Autodesk Inventor part; units mm, degrees
ref_plane "YZ Plane" through (0, 0, 0) normal (1, 0, 0) x (0, 1, 0)
ref_plane "XZ Plane" through (0, 0, 0) normal (0, 1, 0) x (-1, 0, 0)
ref_plane "XY Plane" through (0, 0, 0) normal (0, 0, 1) x (1, 0, 0)
sketch "Sketch1" plane through (0, 0, 0) normal (0, 0, 1) x (1, 0, 0)
  line L0 (-22, 15) -> (-22, 8)
  line L1 (-21, 16) -> (-22, 15)
  line L2 (-12, 16) -> (-21, 16)
  line L3 (-11.8, 15.8) -> (-12, 16)
  arc A0 (-11.8, 15.8) -> (-11.0859, 15.5) centre (-11.0859, 16.5) ccw
  line L4 (-4.9141, 15.5) -> (-11.0859, 15.5)
  arc A1 (-4.9141, 15.5) -> (-4.2, 15.8) centre (-4.9141, 16.5) ccw
  line L5 (-4, 16) -> (-4.2, 15.8)
  line L6 (4, 16) -> (-4, 16)
  line L7 (4.2, 15.8) -> (4, 16)
  arc A2 (4.2, 15.8) -> (4.9141, 15.5) centre (4.9141, 16.5) ccw
  line L8 (11.0859, 15.5) -> (4.9141, 15.5)
  arc A3 (11.0859, 15.5) -> (11.8, 15.8) centre (11.0859, 16.5) ccw
  line L9 (12, 16) -> (11.8, 15.8)
  line L10 (21, 16) -> (12, 16)
  line L11 (22, 15) -> (21, 16)
  line L12 (22, 3) -> (22, 15)
  line L13 (21.5, 2.5) -> (22, 3)
  line L14 (21.5, -8) -> (21.5, 2.5)
  line L15 (20, -9.5) -> (21.5, -8)
  line L16 (9.45, -9.5) -> (20, -9.5)
  line L17 (6.6, -6.65) -> (9.45, -9.5)
  line L18 (6.6, -4.35) -> (6.6, -6.65)
  line L19 (7.7, -3.25) -> (6.6, -4.35)
  arc A4 (9.6, -1.075) -> (7.7, -3.25) centre (9.8292, -3.1926) ccw
  line L20 (10, -0.675) -> (9.6, -1.075)
  line L21 (10, 0.675) -> (10, -0.675)
  line L22 (9.6, 1.075) -> (10, 0.675)
  arc A5 (7.7, 3.1) -> (9.6, 1.075) centre (9.828, 3.1928) ccw
  line L23 (7.3, 3.5) -> (7.7, 3.1)
  line L24 (-7.3, 3.5) -> (7.3, 3.5)
  line L25 (-7.7, 3.1) -> (-7.3, 3.5)
  arc A6 (-9.6, 1.075) -> (-7.7, 3.1) centre (-9.828, 3.1928) ccw
  line L26 (-10, 0.675) -> (-9.6, 1.075)
  line L27 (-10, -0.675) -> (-10, 0.675)
  line L28 (-9.6, -1.075) -> (-10, -0.675)
  arc A7 (-7.7, -3.25) -> (-9.6, -1.075) centre (-9.8292, -3.1926) ccw
  line L29 (-6.6, -4.35) -> (-7.7, -3.25)
  line L30 (-6.6, -6.65) -> (-6.6, -4.35)
  line L31 (-9.45, -9.5) -> (-6.6, -6.65)
  line L32 (-20, -9.5) -> (-9.45, -9.5)
  line L33 (-21.5, -8) -> (-20, -9.5)
  line L34 (-21.5, 7.5) -> (-21.5, -8)
  line L35 (-22, 8) -> (-21.5, 7.5)
  point P0 (0, 0)
  point P1 (0, 0)
extrude "Extrusion1" add sketch "Sketch1" against normal blind 50.5
sketch "Sketch3" plane through (-21, 16, 0) normal (0, 1, 0) x (1, 0, 0)
  circle A0 centre (5.5, 41) radius 2.1
  circle A1 centre (36.5, 41) radius 2.1
  line L0 (9, 0) -> (0, 0)
  line L1 (9, 0) -> (9, 50.5)
  line L2 (0, 50.5) -> (9, 50.5)
  line L3 (0, 0) -> (0, 50.5)
  line L4 (42, 0) -> (33, 0)
  line L5 (42, 0) -> (42, 50.5)
  line L6 (33, 50.5) -> (42, 50.5)
  line L7 (33, 0) -> (33, 50.5)
  line L8 (42, 0) -> (33, 0)
  line L9 (4.5, 0) -> (4.5, 50.5) construction
  line L10 (0, 50.5) -> (9, 50.5)
  line L11 (0, 0) -> (0, 50.5)
  line L12 (0, 25.25) -> (42, 25.25) construction
  line L13 (42, 0) -> (42, 50.5)
  line L14 (21, 0) -> (21, 50.5) construction
  circle A2 centre (5.5, 9.5) radius 2.1
  circle A3 centre (36.5, 9.5) radius 2.1
  point P0 (19, 27.5)
  dimension "d5" = 31
  dimension "d6" = 4.2
  dimension "d7" = 15.75
extrude "Extrusion2" cut sketch "Sketch3" against normal blind 6 contours A0 | A1 | A2 | A3
properties part number "HGR20A"
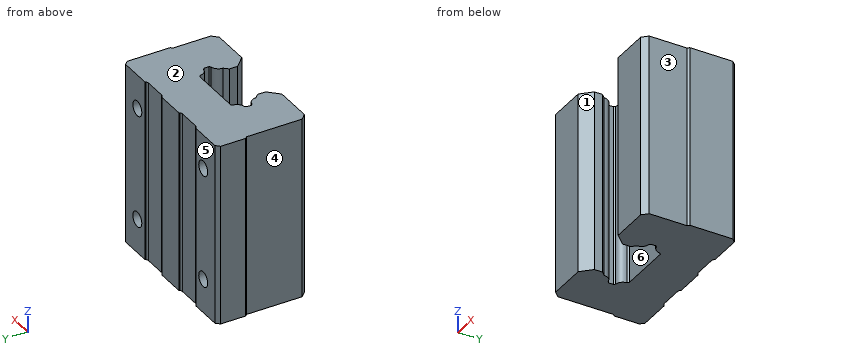
CAD build for the part. Positions are in the model's coordinates, mm. Face numbers are marked on the shaded views. A direction names the side the tool comes from. Give positions to 0.01 mm unless a question says otherwise; leave off trailing zeros. Order: outer loops, then holes, each group sorted by start corner. A loop starts at its lowest first (then second) coordinate and runs counter-clockwise, first axis right, second up.
(1) Flat gauge pins, fed straight in: pin 1 (1.5 mm diameter, centred on y = 0, z = -30.5, fed in from +X); pin 2 (12 mm diameter, centred on x = 4, y = -2.5, fed in from -Z); pin 3 (2 mm diameter, centred on x = -15, z = -9.5, fed in from +Y); pin 4 (11.5 mm diameter, centred on y = -3, z = -20, fed in from +X). Where does each tip first touch, or does it go through?
(2) Tool access for the marked faces 1, 2 and 3: list every direction of +Z, -Z, +X, -X, +Y, -Y with a clear straight run to the whole face (end or side of a thin tool).
(3) Saw through at B-B, the plane x = 15.5. Give the cut face in (y, z), then the cut area to 3 significant figures.
(4) Mould opens along X. For the marked faces 4, 5 and 6 say: released by +X, released by -X, zero draft, split by the parting line, or undercut.
(5) Saw through at A-A, the plane y = 14.25. Give the cut face in (x, z), then the cut area to 3 significant figures.
(6) Drill centre lines: L1, parallel to Z at x = 15.5, y = 13.05; L2, parallel to X at y = 14.55, z = -9.5; L3, parallel to X at y = -6.25, z = -8. Where is each one in solid material? Low to high.
Results found:
1. pin 1: stops at x = 21.5
1. pin 2: stops at z = -50.5
1. pin 3: stops at y = 10
1. pin 4: stops at x = 21.75
2. face 1: +Z, -Z, -Y
2. face 2: +Z, +X, -X, +Y, -Y
2. face 3: +Z, -Z, +X, -Y
3. outline: (-9.5, -50.5) - (16, -50.5) - (16, -43.1) - (10, -43.1) - (10, -38.9) - (16, -38.9) - (16, -11.6) - (10, -11.6) - (10, -7.4) - (16, -7.4) - (16, 0) - (-9.5, 0) - close
3. area: 1,240 mm2
4. face 4: released by -X
4. face 5: zero draft
4. face 6: undercut
5. outline: (-22, -50.5) - (22, -50.5) - (22, 0) - (-22, 0) - close; hole circle Ø4.2 at (-15.5, -41); hole circle Ø4.2 at (-15.5, -9.5); hole circle Ø4.2 at (15.5, -41); hole circle Ø4.2 at (15.5, -9.5)
5. area: 2,170 mm2
6. L1: z = -50.5 to -43.1, -38.9 to -11.6, -7.4 to 0
6. L2: x = -22 to -17.6, -13.4 to 13.4, 17.6 to 22
6. L3: x = -21.5 to -6.6, 6.6 to 21.5
